CAD build for the part. Positions are in the model's coordinates, mm. A direction names the side the tool comes from. Round coordinates to 2 decimals unless told otherwise and drop trailing zeros. Loops run counter-clockwise (first coordinate to the right, second up) from the corner with the lowest first, then second, coordinate; pieces in that order, holes last. Notation, with made-up numbers: (-27.5, -31.75) - (13.5, -31.75) arc R23 cw to (13.5, 6.25) - close; hole circle Ø6 at (-29.5, 49.25). An arc over 180 degrees is marked (long way). Use one line per item in the form item = value.
from build123d import *

# Parameters (mm, degrees)
SKETCH2_R           = 16
SKETCH2_R_2         = 8
BOSS_EXTRUDE1_DEPTH = 56
BOSS_EXTRUDE2_DEPTH = 28
SKETCH4_R           = 8
CUT_EXTRUDE1_DEPTH  = 28
SKETCH5_R           = 8
CUT_EXTRUDE2_DEPTH  = 56


with BuildPart() as part:
    # Sketch2 → Boss-Extrude1 (new body)
    with BuildSketch(Plane.XY):
        Circle(SKETCH2_R)
        Circle(SKETCH2_R_2, mode=Mode.SUBTRACT)
    extrude(amount=BOSS_EXTRUDE1_DEPTH)

    # Sketch3 → Boss-Extrude2 (add, symmetric)
    with BuildSketch(Plane(origin=(0, 0, 0), x_dir=(0, 0, -1), z_dir=(1, 0, 0))):
        with BuildLine():
            ThreePointArc((-44, 18), (-28, 2), (-12, 18))
            Line((-12, 18), (-20, 18))
            ThreePointArc((-20, 18), (-28, 10), (-36, 18))
            Line((-36, 18), (-44, 18))
        make_face()
        with BuildLine():
            Line((-20, 18), (-12, 18))
            ThreePointArc((-12, 18), (-28, 34), (-44, 18))
            Line((-44, 18), (-36, 18))
            ThreePointArc((-36, 18), (-28, 26), (-20, 18))
        make_face()
        with BuildLine():
            ThreePointArc((-44, 18), (-28, 2), (-12, 18))
            Line((-12, 18), (-20, 18))
            ThreePointArc((-20, 18), (-28, 10), (-36, 18))
            Line((-36, 18), (-44, 18))
        make_face()
        with BuildLine():
            Line((-20, 18), (-12, 18))
            ThreePointArc((-12, 18), (-28, 34), (-44, 18))
            Line((-44, 18), (-36, 18))
            ThreePointArc((-36, 18), (-28, 26), (-20, 18))
        make_face()
    extrude(amount=BOSS_EXTRUDE2_DEPTH, both=True)

    # Sketch4 → Cut-Extrude1 (cut, symmetric)
    with BuildSketch(Plane(origin=(0, 0, 0), x_dir=(0, 0, -1), z_dir=(1, 0, 0))):
        with Locations((-28, 18)):
            Circle(SKETCH4_R)
    extrude(amount=CUT_EXTRUDE1_DEPTH, both=True, mode=Mode.SUBTRACT)

    # Sketch5 → Cut-Extrude2 (cut)
    with BuildSketch(Plane.XY):
        Circle(SKETCH5_R)
    extrude(amount=CUT_EXTRUDE2_DEPTH, mode=Mode.SUBTRACT)


solid = part.part
1) Slice it at B-B (z = 24). Write the cut outline in (x, y).
Report:
outline = (-28, 2.51) - (-15.8, 2.51) arc R16 ccw (long way) to (15.8, 2.51) - (28, 2.51) - (28, 11.07) - (-28, 11.07) - close; (-28, 24.93) - (28, 24.93) - (28, 33.49) - (-28, 33.49) - close; hole circle Ø16 at (0, 0)
2) Drill centre lines: probe 1 along Y at (x, z) = (0, 28); probe 2 along Y at (x, z) = (0, 23) (3 decimals); probe 3 along Y at (x, z) = (0, 13.5). Where is each one in solid material? Low to high.
Report:
probe_1 = -16 to -8, 8 to 10, 26 to 34
probe_2 = -16 to -8, 8 to 11.755, 24.245 to 33.199
probe_3 = -16 to -8, 8 to 24.76
3) Flat gauge pins, fed straight in: pin 1 (4 mm diameter, centred on x = -11.5, z = 44.5, fed in from +Y); pin 2 (12 mm diameter, centred on y = 27.5, z = 49.5, fed in from -X); pin 3 (1 mm diameter, centred on x = 10, z = 14.5, fed in from +Y); pin 4 (8 mm diameter, centred on x = 10, z = 9, fed in from -Y). Where does each tip first touch, or does it go through?
Report:
pin_1 = 24.76
pin_2 = through
pin_3 = 27.33
pin_4 = -14.83
4) Slice it at C-C (x = -5.5). Write the cut outline in (y, z).
Report:
outline = (-15.02, 0) - (-5.81, 0) - (-5.81, 56) - (-15.02, 56) - close; (5.81, 0) - (15.02, 0) - (15.02, 12.28) arc R16 ccw (long way) to (15.02, 43.72) - (15.02, 56) - (5.81, 56) - close; hole circle Ø16 at (18, 28)
5) Slice it at A-A (y = 18). Write the cut outline in (x, z), plus the area to 3 significant figures.
Report:
outline = (-28, 12) - (28, 12) - (28, 20) - (-28, 20) - close; (-28, 36) - (28, 36) - (28, 44) - (-28, 44) - close
area = 896 mm^2
6) Tool access for faces 1 (the flat face through (-3.8, 7.3, 56)), 2 (the cylindrical face through (-3.47, -15.62, 27.61)): list every direction of +Z, -Z, +X, -X, +Y, -Y with a clear straight run to the whole face (end or side of a thin tool).
Report:
face_1 = +Z, +X, -X, +Y, -Y
face_2 = none
7) Slice it at D-D (z = 17). Write the cut outline in (x, y).
Report:
outline = (-28, 6.38) - (-14.67, 6.38) arc R16 ccw (long way) to (14.67, 6.38) - (28, 6.38) - (28, 29.62) - (-28, 29.62) - close; hole circle Ø16 at (0, 0)
